from build123d import *

# Parameters (mm, degrees)
SKETCH1_W            = 125
SKETCH1_H            = 135
BOSS_EXTRUDE1_DEPTH  = 5
SKETCH2_W            = 5
SKETCH2_H            = 135
BOSS_EXTRUDE2_DEPTH  = 51.5
SKETCH3_W            = 5
SKETCH3_H            = 135
BOSS_EXTRUDE3_DEPTH  = 51.5
SKETCH5_W            = 115
SKETCH5_H            = 7.57
BOSS_EXTRUDE4_DEPTH  = 51.5
SKETCH21_W           = 2.5
SKETCH21_H           = 55
BOSS_EXTRUDE13_DEPTH = 46.5
SKETCH23_W           = 115
SKETCH23_H           = 2.5
BOSS_EXTRUDE14_DEPTH = 25
BOSS_EXTRUDE15_REACH = 177.789
SKETCH24_W           = 35
SKETCH24_H           = 1.5
SKETCH25_W           = 80
SKETCH25_H           = 2.5
BOSS_EXTRUDE16_DEPTH = 26.5
SKETCH27_W           = 2.5
SKETCH27_H           = 28
BOSS_EXTRUDE20_DEPTH = 104.93
CUT_EXTRUDE1_REACH   = 188.414
SKETCH28_W           = 35
SKETCH28_H           = 55
SKETCH29_W           = 80
SKETCH29_H           = 5
CUT_EXTRUDE2_DEPTH   = 178.363341477
SKETCH35_W           = 20
SKETCH35_H           = 15
CUT_EXTRUDE5_DEPTH   = 7.5


with BuildPart() as part:
    # Sketch1 → Boss-Extrude1 (new body)
    with BuildSketch(Plane.XY):
        with Locations((62.5, 67.5)):
            Rectangle(SKETCH1_W, SKETCH1_H)
    extrude(amount=BOSS_EXTRUDE1_DEPTH)

    # Sketch2 → Boss-Extrude2 (add)
    with BuildSketch(Plane.XY.offset(5)):
        with Locations((2.5, 67.5)):
            Rectangle(SKETCH2_W, SKETCH2_H)
    extrude(amount=BOSS_EXTRUDE2_DEPTH)

    # Sketch3 → Boss-Extrude3 (add)
    with BuildSketch(Plane.XY.offset(5)):
        with Locations((122.5, 67.5)):
            Rectangle(SKETCH3_W, SKETCH3_H)
    extrude(amount=BOSS_EXTRUDE3_DEPTH)

    # Sketch5 → Boss-Extrude4 (add)
    with BuildSketch(Plane.XY.offset(5)):
        with Locations((62.5, 3.785)):
            Rectangle(SKETCH5_W, SKETCH5_H)
    extrude(amount=BOSS_EXTRUDE4_DEPTH)

    # Sketch21 → Boss-Extrude13 (add)
    with BuildSketch(Plane.XY.offset(5)):
        with Locations((41.25, 102.5)):
            Rectangle(SKETCH21_W, SKETCH21_H)
    extrude(amount=BOSS_EXTRUDE13_DEPTH)

    # Sketch23 → Boss-Extrude14 (add)
    with BuildSketch(Plane.XY.offset(5)):
        with Locations((62.5, 23.82)):
            Rectangle(SKETCH23_W, SKETCH23_H)
    extrude(amount=BOSS_EXTRUDE14_DEPTH)

    # Boss-Extrude15: up to this face of the body (flat: up to its plane)
    boss_extrude15_end = Plane(part.part.faces().sort_by_distance((41.25, 130, 28.25))[0])
    # Sketch24 → Boss-Extrude15 (add, up to the picked face)
    with BuildSketch(Plane(origin=(0, 25.07, 0), x_dir=(1, 0, 0), z_dir=(0, 1, 0)), mode=Mode.PRIVATE) as boss_extrude15_sk1:
        with Locations((22.5, -29.25)):
            Rectangle(SKETCH24_W, SKETCH24_H)
    boss_extrude15_tool1 = split(extrude(boss_extrude15_sk1.sketch, amount=BOSS_EXTRUDE15_REACH, mode=Mode.PRIVATE), bisect_by=boss_extrude15_end, keep=Keep.BOTH, mode=Mode.PRIVATE)
    add(boss_extrude15_tool1.solids().sort_by(Axis((22.5, 25.07, 29.25), (0, 1, 0)))[0])

    # Sketch25 → Boss-Extrude16 (add)
    with BuildSketch(Plane.XY.offset(30)):
        with Locations((80, 23.82)):
            Rectangle(SKETCH25_W, SKETCH25_H)
    extrude(amount=BOSS_EXTRUDE16_DEPTH)

    # Sketch27 → Boss-Extrude20 (add)
    with BuildSketch(Plane(origin=(0, 25.07, 0), x_dir=(1, 0, 0), z_dir=(0, 1, 0))):
        with Locations((41.25, -42.5)):
            Rectangle(SKETCH27_W, SKETCH27_H)
    extrude(amount=BOSS_EXTRUDE20_DEPTH)

    # Sketch28 → Cut-Extrude1 (cut, up to next)
    with BuildSketch(Plane.XY.offset(30), mode=Mode.PRIVATE) as cut_extrude1_sk1:
        with Locations((22.5, 102.5)):
            Rectangle(SKETCH28_W, SKETCH28_H)
    cut_extrude1_tool1 = extrude(cut_extrude1_sk1.sketch, amount=-CUT_EXTRUDE1_REACH, mode=Mode.PRIVATE) & part.part
    add(cut_extrude1_tool1.solids().sort_by_distance((22.5, 102.5, 30))[0], mode=Mode.SUBTRACT)

    # Sketch29 → Cut-Extrude2 (cut, through all)
    with BuildSketch(Plane.XZ.offset(-22.57)):
        with Locations((80, 54)):
            Rectangle(SKETCH29_W, SKETCH29_H)
    extrude(amount=-CUT_EXTRUDE2_DEPTH, mode=Mode.SUBTRACT)

    # Sketch35 → Cut-Extrude5 (cut)
    with BuildSketch(Plane(origin=(125, 0, 0), x_dir=(0, 0, -1), z_dir=(1, 0, 0))):
        with Locations((-41.5, 15.07)):
            Rectangle(SKETCH35_W, SKETCH35_H)
    extrude(amount=-CUT_EXTRUDE5_DEPTH, mode=Mode.SUBTRACT)


solid = part.part
Design review of the part built by this model. Coordinates are the model's own, in mm. A direction names the side the tool comes from. Round coordinates to 2 decimals unless told otherwise and drop trailing zeros. Write each loop counter-clockwise with the first axis right and the second up, starting at its lowest first coordinate (ties: lowest second). Pieces come first, ordered by that corner, then holes. Notation, with made-up numbers: (53, 59) - (96, 59) arc R16 ccw to (96, 63) - close; hole circle Ø11 at (61.5, 89.5). An arc over 180 degrees is marked (long way). Use a Markdown table: item, result. Add a question column.
1. Clearance check with flat-ended pins moving along their axes: pin 1 (2 mm diameter, centred on x = 61.5, z = 11, fed in from +Y); pin 2 (8 mm diameter, centred on x = 76.5, y = 64.5, fed in from +Z); pin 3 (3 mm diameter, centred on x = 39.5, z = 21, fed in from +Y). State where each tip first meets the part, or that it passes through.
2. We need section A-A (z = 16). State the section outline as (x, y) points.
3. Mouldability with a two-part tool opening along Y and no side actions: class faces 4 (the face through (77, 22.57, 28)), 5 (the face through (58, 135, 3)), 6 (the face through (41, 52, 51.5)) as +Y half, -Y half, draft (parallel to the pull), parting line (faces both ways), or undercut.
4. We need section D-D (z = 37). State the section outline as (x, y) points, then the cut area to 3 significant figures.
5. We need section C-C (x = 31). State the section outline as (y, z) points.
6. For faces 1 (the face through (40, 87, 34)), 2 (the face through (123, 15, 31.5)), 3 (the face through (120, 15, 18)), list the 3-axis set-ups (+Z, -Z, +X, -X, +Y, -Y) from which the entire face can be reached by the end or side of a thin tool; tool diameter is ignored.
7. We need section B-B (y = 124.5). State the section outline as (x, z) points, then the cut area to 3 significant figures.
8. Wall thickness on probe 1 along X at (y, z) = (41.5, 36.5); probe 2 along X at (y, z) = (31, 7.5); probe 3 along Y at (x, z) = (52, 20): over which ranges is each line inside the solid? List them lowest first.
Output:
| question | item | result |
|---|---|---|
| 1 | pin 1 | stops at y = 25.07 |
| 1 | pin 2 | stops at z = 5 |
| 1 | pin 3 | stops at y = 130 |
| 2 | outline | (0, 0) - (125, 0) - (125, 135) - (120, 135) - (120, 25.07) - (5, 25.07) - (5, 135) - (0, 135) - close; (40, 75) - (42.5, 75) - (42.5, 130) - (40, 130) - close; hole (5, 7.57) - (120, 7.57) - (120, 22.57) - (5, 22.57) - close |
| 3 | face 4 | undercut |
| 3 | face 5 | +Y half |
| 3 | face 6 | draft |
| 4 | outline | (0, 0) - (125, 0) - (125, 7.57) - (5, 7.57) - (5, 135) - (0, 135) - close; (40, 22.57) - (125, 22.57) - (125, 135) - (120, 135) - (120, 25.07) - (42.5, 25.07) - (42.5, 130) - (40, 130) - close |
| 4 | area | 2,610 mm2 |
| 5 | outline | (0, 0) - (135, 0) - (135, 5) - (25.07, 5) - (25.07, 28.5) - (75, 28.5) - (75, 30) - (22.57, 30) - (22.57, 5) - (7.57, 5) - (7.57, 56.5) - (0, 56.5) - close |
| 6 | face 1 | +Z, +Y |
| 6 | face 2 | +X |
| 6 | face 3 | +Z |
| 7 | outline | (0, 0) - (125, 0) - (125, 56.5) - (120, 56.5) - (120, 5) - (42.5, 5) - (42.5, 51.5) - (40, 51.5) - (40, 5) - (5, 5) - (5, 56.5) - (0, 56.5) - close |
| 7 | area | 1,260 mm2 |
| 8 | probe 1 | x = 0 to 5, 40 to 42.5, 120 to 125 |
| 8 | probe 2 | x = 0 to 5, 120 to 125 |
| 8 | probe 3 | y = 0 to 7.57, 22.57 to 25.07 |
